Input: dimensioned drawing with shaded views. Units: mm. Origin: part minimum x, y, z. A direction names the side the tool comes from. Round coordinates to 2 decimals unless told otherwise and drop trailing zeros. Order: outer loops, then holes, each group sorted by start corner. A loop starts at its lowest first (then second) coordinate and runs counter-clockwise, first axis right, second up. Notation, with made-up numbers: (79.25, 74) - (101.25, 74) arc R32 cw to (101.25, 108) - close; hole circle Ø7 at (27, 21). An arc over 180 degrees is marked (long way). One line per item, written item: value. Start each with the question number.
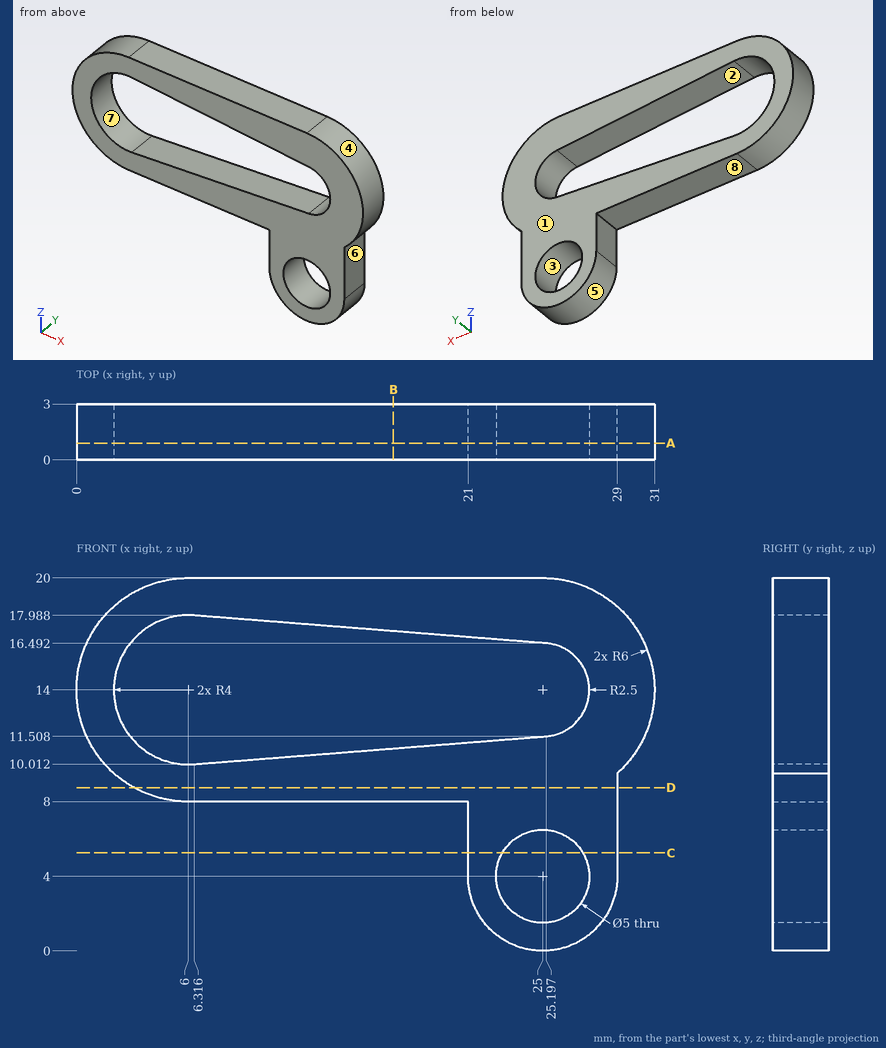
1. Pin query (flat end, axial travel): pin 1 (0.9 mm diameter, centred on y = 1, z = 7.5, fed in from +X). Return the tip coordinate at first contact, or that it passes through.
2. Line query: line 1 (X direction, y = 1.1, z = 4); line 2 (Z direction, x = 23.5, y = 1.45) (1 decimal); line 3 (Z direction, x = 27, y = 0.9) (1 decimal). Output: solid intervals per line, ascending. Write a range as from..to.
3. Section D-D (z = 8.75). Return the cut outline in (x, y) (1 decimal).
4. Section C-C (z = 5.25). Return the cut outline in (x, y) (1 decimal).
5. Pull-direction query (Z, two-part tool) for the marked faces 1, 2, 3 and 4; classes: released by +Z, released by -Z, zero draft, split by the parting line, or undercut.
6. Section A-A (y = 0.9). Return the cut outline in (x, z) (1 decimal).
7. Set-up query: the marked faces 5, 6, 7 and 8. Return all of +Z, -Z, +X, -X, +Y, -Y with unobstructed straight access to the full face (end or side cutting, diameter ignored); none if empty.
8. Section B-B (x = 17). Return the cut outline in (y, z).
Solved:
1. pin 1: stops at x = 29
2. line 1: x = 21..22.5, 27.5..29
2. line 2: z = 0.3..2, 6..11.4, 16.6..20
2. line 3: z = 0.5..2.5, 5.5..12.5, 15.5..19.7
3. outline: (3.1, 0) - (29, 0) - (29, 3) - (3.1, 3) - close
4. outline: (21, 0) - (22.8, 0) - (22.8, 3) - (21, 3) - close; (27.2, 0) - (29, 0) - (29, 3) - (27.2, 3) - close
5. face 1: zero draft
5. face 2: undercut
5. face 3: undercut
5. face 4: split by the parting line
6. outline: (6, 8) - (21, 8) - (21, 4) arc R4 ccw to (29, 4) - (29, 9.5) arc R6 ccw to (25, 20) - (6, 20) arc R6 ccw to start; hole (6.3, 10) - (25.2, 11.5) arc R2.5 ccw to (25.2, 16.5) - (6.3, 18) arc R4 ccw (long way) to start; hole circle Ø5 at (25, 4)
7. face 5: -Z, +Y, -Y
7. face 6: -Z, +X, +Y, -Y
7. face 7: +Y, -Y
7. face 8: -Z, -X, +Y, -Y
8. outline: (0, 8) - (3, 8) - (3, 10.86) - (0, 10.86) - close; (0, 17.14) - (3, 17.14) - (3, 20) - (0, 20) - close
